Geometry: final body of the model. Coordinates: model frame, mm. Face numbers are marked on the shaded views. A direction names the side the tool comes from. Give positions to 0.01 mm unless a question says otherwise; leave off trailing zeros. Write each loop counter-clockwise with the first axis right and the second up, starting at its lowest first coordinate (ties: lowest second). Pieces come first, ordered by that corner, then holes.
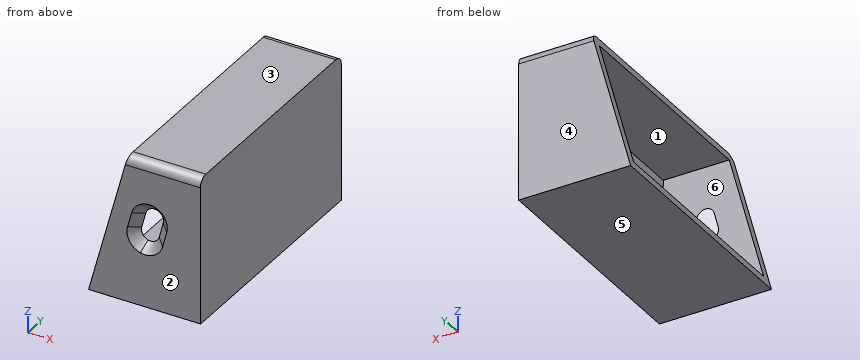
Autodesk Fusion 360 part; units mm, degrees
sketch "Sketch1" plane through (0, 0, 0) normal (0, 1, 0) x (1, 0, 0)
  line L0 (0, 0) -> (24, 0)
  line L1 (0, 0) -> (12.941, -48.2963)
  line L2 (0, 0) -> (50, 0) construction
  line L3 (24, 0) -> (36.941, -48.2963)
  line L4 (24, 0) -> (74, 0) construction
  line L5 (12.941, -48.2963) -> (36.941, -48.2963)
  line L6 (36.941, -48.2963) -> (37, 0)
  line L7 (24, 0) -> (37, 0)
  dimension "d1" = 24
  dimension "d2" = 75
  dimension "d3" = 50
  dimension "d4" = 50
  dimension "d5" = 75
extrude "Extrude1" add sketch "Sketch1" along normal blind 78.5
shell "Shell1" thickness 3 removed faces 1 at (4.3137, 26.1667, 16.0988)
sketch "Sketch2" plane through (0, 0, 0) normal (0, -1, 0) x (1, 0, 0)
  line L0 (12.941, 48.2963) -> (0, 0)
  line L1 (0, 0) -> (37, 0)
  line L2 (36.941, 48.2963) -> (12.941, 48.2963)
  line L3 (17.8998, 20.4386) -> (17.8858, 20.4424)
  line L4 (21.5638, 22.5776) -> (22.8982, 27.6553)
  line L5 (20.7731, 31.3156) -> (20.8115, 31.3053)
  line L6 (17.1373, 29.184) -> (15.7785, 24.1128)
  arc A0 (20.8115, 31.3053) -> (17.1373, 29.184) centre (20.0351, 28.4075) ccw
  arc A1 (15.7785, 24.1128) -> (17.8998, 20.4386) centre (18.6763, 23.3364) ccw
  arc A2 (17.8858, 20.4424) -> (21.5638, 22.5776) centre (18.6623, 23.3401) ccw
  arc A3 (22.8982, 27.6553) -> (20.7731, 31.3156) centre (19.9967, 28.4178) ccw
  line L7 (37, 0) -> (36.941, 48.2963)
  point P0 (15.002, 21.2151)
  point P1 (20.7976, 19.6622)
  point P2 (17.9138, 32.0817)
  dimension "d9" = 6
  dimension "d10" = 11.25
  dimension "d11" = 9
  dimension "d12" = 24.375
  dimension "d13" = 3
extrude "Extrude2" cut sketch "Sketch2" against normal blind 18 contours L3 L4 L5 L6 A0 A1 A2 A3
chamfer "Chamfer1" distance 3 angle 45 6 edges at (20.1717, 0, 20.7475) (22.231, 0, 25.1165) (22.5961, 0, 29.9154) (16.4579, 0, 26.6484) (16.0764, 0, 21.8395) (18.5265, 0, 31.0006)
fillet "Fillet1" radius 3 2 edges at (24.941, 0, 48.2963) (24.941, 78.5, 48.2963)
equation "d12 = 30 mm - ( 11.25 / 2 ) * 1 mm"
Q1. Section B-B on y = 24.5. Output: boundary loops of the cut face in (x, z).
Filled sheet:
outline: (0, 0) - (37, 0) - (36.94, 48.3) - (12.94, 48.3) - (12.14, 45.3) - (33.94, 45.3) - (34, 3) - (0.8, 3) - close
Q2. Section C-C on z = 10. Output: boundary loops of the cut face in (x, y), plus the area to 3 significant figures.
Filled sheet:
outline: (2.68, 0) - (36.99, 0) - (36.99, 78.5) - (2.68, 78.5) - (2.68, 75.5) - (33.99, 75.5) - (33.99, 3) - (2.68, 3) - close
area: 423 mm2
Q3. Pin query (flat end, axial travel): P1, Ø8, axis at y = 52, z = 18, coming from the -X side; P2, Ø2, axis at y = 32.5, z = 24.5, coming from the +X side. Return the tip coordinate at first contact, or that it passes through.
Filled sheet:
P1: stops at x = 33.97
P2: stops at x = 36.97
Q4. Ray query, line 1 along Y through (x, z) = (3, 8.5); line 2 along Z through (x, y) = (13, 51); line 3 along Y through (x, z) = (16.5, 25). Return the intervals inside material, ascending.
Filled sheet:
line 1: y = 0 to 3, 75.5 to 78.5
line 2: z = 0 to 3, 45.3 to 48.3
line 3: y = 75.5 to 78.5
Q5. Section A-A on x = 33. Output: boundary loops of the cut face in (y, z).
Filled sheet:
outline: (0, 0) - (78.5, 0) - (78.5, 45.3) arc R3 ccw to (75.5, 48.3) - (3, 48.3) arc R3 ccw to (0, 45.3) - close; hole (3, 3) - (75.5, 3) - (75.5, 45.3) - (3, 45.3) - close
Q6. Access query for the marked faces 5 and 6. Directions: +Z, -Z, +X, -X, +Y, -Y. A direction counts if a zero-diameter tool reaches every point of the face in a straight line with its end or side. Return the directions, or none.
Filled sheet:
face 5: -Z, +X, -X, +Y, -Y
face 6: -X
Q7. Pull-direction query (Y, two-part tool) for the marked faces 1, 2, 3 and 4; classes: released by +Y, released by -Y, zero draft, split by the parting line, or undercut.
Filled sheet:
face 1: undercut
face 2: released by -Y
face 3: zero draft
face 4: released by +Y
